Input: part model. Units: mm. Frame: model coordinates. Face numbers are marked on the shaded views. A direction names the side the tool comes from. Round coordinates to 2 decimals unless told otherwise and drop trailing zeros. Loops run counter-clockwise (first coordinate to the right, second up) from the corner with the lowest first, then second, coordinate; pieces in that order, holes last. Notation, with made-up numbers: (18, -21.75) -> (57, -21.75) arc R16 ccw to (57, -2.75) -> close; hole circle Ø5 at (78, -1). An arc over 180 degrees is marked (long way). Answer as a JSON object with one key per item and string values.
```python
from build123d import *

# Parameters (mm, degrees)
SKETCH1_R               = 7
SKETCH1_R_2             = 4.05
BOSS_EXTRUDE1_DEPTH     = 15
BOSS_EXTRUDE2_START     = -15
SKETCH1_3_R             = 7
SKETCH1_3_R_2           = 4.05
SKETCH1_3_R_3           = 1.7
BOSS_EXTRUDE2_DEPTH     = 15
SKETCH3_W               = 6
SKETCH3_H               = 3
CUT_EXTRUDE2_DEPTH      = 11
BOSS_EXTRUDE3_DEPTH     = 11
BOSS_EXTRUDE4_START     = -11
BOSS_EXTRUDE4_DEPTH     = 11
CUT_EXTRUDE1_DEPTH      = 20.874606914
CUT_EXTRUDE1_DEPTH_BACK = 20.874606914
SKETCH2_R               = 1.5


with BuildPart() as part:
    # Sketch1 → Boss-Extrude1 (new body)
    with BuildSketch(Plane(origin=(0, 0, 0), x_dir=(1, 0, 0), z_dir=(0, 1, 0))):
        with Locations(Location((0, 0, 0), (0, 0, 270))):
            Circle(SKETCH1_R)
        with Locations(Location((0, 0, 0), (0, 0, 270))):
            Circle(SKETCH1_R_2, mode=Mode.SUBTRACT)
    extrude(amount=BOSS_EXTRUDE1_DEPTH)

    # Sketch1_3 → Boss-Extrude2 (add)
    # profile 1 of 2: a face of its own
    with BuildSketch(Plane(origin=(0, 0, 0), x_dir=(1, 0, 0), z_dir=(0, 1, 0)).offset(BOSS_EXTRUDE2_START)):
        with Locations(Location((0, 0, 0), (0, 0, 270))):
            Circle(SKETCH1_3_R)
        with Locations(Location((0, 0, 0), (0, 0, 270))):
            Circle(SKETCH1_3_R_2, mode=Mode.SUBTRACT)
    # profile 2 of 2: a face of its own
    with BuildSketch(Plane(origin=(0, 0, 0), x_dir=(1, 0, 0), z_dir=(0, 1, 0)).offset(BOSS_EXTRUDE2_START)):
        with Locations(Location((0, 0, 0), (0, 0, 270))):
            Circle(SKETCH1_3_R_2)
        with Locations(Location((0, 0, 0), (0, 0, 270))):
            Circle(SKETCH1_3_R_3, mode=Mode.SUBTRACT)
    extrude(amount=BOSS_EXTRUDE2_DEPTH)

    # Sketch3 → Cut-Extrude2 (cut)
    with BuildSketch(Plane.XZ.offset(15)):
        with Locations((0, 5)):
            Rectangle(SKETCH3_W, SKETCH3_H)
    extrude(amount=-CUT_EXTRUDE2_DEPTH, mode=Mode.SUBTRACT)

    # Sketch3_3 → Boss-Extrude3 (add)
    with BuildSketch(Plane.XZ.offset(15)):
        with BuildLine():
            Line((-3, 6.32455532), (-3, 6.5))
            Line((-3, 6.5), (-2.598076211, 6.5))
            ThreePointArc((-2.598076211, 6.5), (0, 7), (2.598076211, 6.5))
            Line((2.598076211, 6.5), (3, 6.5))
            Line((3, 6.5), (3, 6.32455532))
            ThreePointArc((3, 6.32455532), (4.063012013, 5.700169593), (5, 4.898979486))
            Line((5, 4.898979486), (5, 8.5))
            Line((5, 8.5), (-5, 8.5))
            Line((-5, 8.5), (-5, 4.898979486))
            ThreePointArc((-5, 4.898979486), (-4.063012013, 5.700169593), (-3, 6.32455532))
        make_face()
    extrude(amount=-BOSS_EXTRUDE3_DEPTH)

    # Sketch4 → Boss-Extrude4 (add)
    with BuildSketch(Plane(origin=(0, 15, 0), x_dir=(1, 0, 0), z_dir=(0, 1, 0)).offset(BOSS_EXTRUDE4_START)):
        with BuildLine():
            Line((-3.605551275, -6), (-3, -6))
            Line((-3, -6), (3, -6))
            Line((3, -6), (3.605551275, -6))
            ThreePointArc((3.605551275, -6), (4.337849667, -5.4939112), (5, -4.898979486))
            Line((5, -4.898979486), (-5, -4.898979486))
            ThreePointArc((-5, -4.898979486), (-4.337849667, -5.4939112), (-3.605551275, -6))
        make_face()
        with BuildLine():
            Line((-3, -9), (-3, -6.32455532))
            ThreePointArc((-3, -6.32455532), (-3.306759887, -6.169711423), (-3.605551275, -6))
            Line((-3.605551275, -6), (-5, -6))
            Line((-5, -6), (-5, -11))
            Line((-5, -11), (5, -11))
            Line((5, -11), (5, -6))
            Line((5, -6), (3.605551275, -6))
            ThreePointArc((3.605551275, -6), (3.306759887, -6.169711423), (3, -6.32455532))
            Line((3, -6.32455532), (3, -9))
            Line((3, -9), (-3, -9))
        make_face()
        with BuildLine():
            Line((-5, -6), (-3.605551275, -6))
            ThreePointArc((-3.605551275, -6), (-4.337849667, -5.4939112), (-5, -4.898979486))
            Line((-5, -4.898979486), (-5, -6))
        make_face()
        with BuildLine():
            ThreePointArc((5, -4.898979486), (4.337849667, -5.4939112), (3.605551275, -6))
            Line((3.605551275, -6), (5, -6))
            Line((5, -6), (5, -4.898979486))
        make_face()
    extrude(amount=BOSS_EXTRUDE4_DEPTH)

    # Sketch2 → Cut-Extrude1 (cut, two sides: drawn at the far end of the back side and taken through both)
    with BuildSketch(Plane.XY.offset(-CUT_EXTRUDE1_DEPTH_BACK)):
        with Locations((0, 8)):
            Circle(SKETCH2_R)
        with Locations(Location((0, -8, 0), (0, 0, 180))):
            Circle(SKETCH2_R)
    extrude(amount=CUT_EXTRUDE1_DEPTH + CUT_EXTRUDE1_DEPTH_BACK, mode=Mode.SUBTRACT)


solid = part.part
```
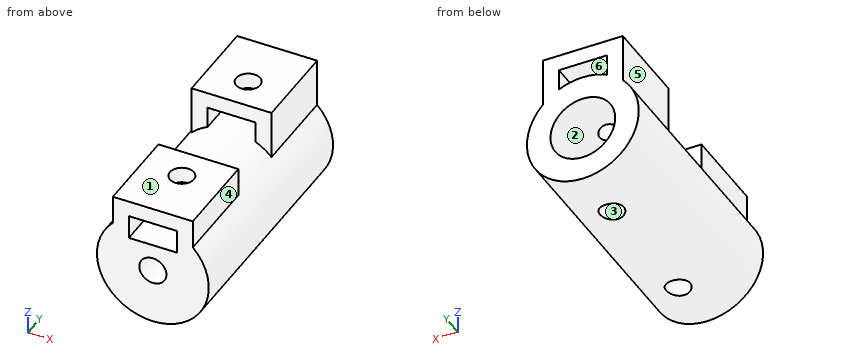
1) Section B-B, the plane z = 3. Output: boundary loops of the cut face in (x, y), plus the area to 3 significant figures.
Output:
{"outline": "(-6.32, -15) -> (6.32, -15) -> (6.32, 15) -> (2.72, 15) -> (2.72, 0) -> (-2.72, 0) -> (-2.72, 15) -> (-6.32, 15) -> close; hole circle Ø3 at (0, -8)", "area": "291 mm^2"}
2) Ray query, probe 1 along Y at (x, z) = (0, -6); probe 2 along X at (y, z) = (-8.5, 6); probe 3 along X at (y, z) = (-4.5, 0). Return the intervals inside material, ascending.
Output:
{"probe 1": "y = -15 to -9.5, -6.5 to 6.5, 9.5 to 15", "probe 2": "x = -5 to -3, 3 to 5", "probe 3": "x = -7 to -1.7, 1.7 to 7"}
3) Section A-A, the plane y = -5.5. Output: boundary loops of the cut face in (x, z), plus the area to 3 significant figures.
Output:
{"outline": "(-5, 4.9) arc R7 ccw (long way) to (5, 4.9) -> (5, 8.5) -> (-5, 8.5) -> close; hole (-3, 3.5) -> (3, 3.5) -> (3, 6.5) -> (-3, 6.5) -> close; hole circle Ø3.4 at (0, 0)", "area": "148 mm^2"}
4) Contact query for flat-ended pins moving along their axis: P1, Ø5, axis at x = -1, y = 11, coming from the -Z side; P2, Ø5, axis at x = -1, y = -9, coming from the +Z side; P3, Ø5, axis at y = 3.5, z = 5, coming from the -X side; P4, Ø1, axis at x = 4, y = 9.5, coming from the -Z side. Output: stop coordinate, or through.
Output:
{"P1": "stops at z = -7", "P2": "stops at z = 8.5", "P3": "stops at x = -6.54", "P4": "stops at z = -6.06"}
5) Section D-D, the plane x = 0. Count the separate pieces of the cut face and the enclosed holes in it, plus the area to 3 significant figures.
Output:
{"separate pieces": "9", "enclosed holes": "0", "area": "202 mm^2"}
6) Reachability of the marked faces 4, 5 and 6 from +Z, -Z, +X, -X, +Y, -Y: full face, straight path, thin tool, end or side. Return the list, or none.
Output:
{"face 4": "+Z, +X, +Y, -Y", "face 5": "+Z, -X, +Y, -Y", "face 6": "+Y, -Y"}
7) Draft query along Z for the marked faces 1, 2 and 3. Return one class per face: +Z half, -Z half, draft (parallel to the pull), parting line (faces both ways), or undercut.
Output:
{"face 1": "+Z half", "face 2": "undercut", "face 3": "draft"}
8) Section C-C, the plane y = 8. Output: boundary loops of the cut face in (x, z), plus the area to 3 significant figures.
Output:
{"outline": "(-5, 4.9) arc R7 ccw to (-1.5, -6.84) -> (-1.5, -3.76) arc R4.05 cw to (-1.5, 3.76) -> (-1.5, 6.84) arc R7 ccw to (-3, 6.32) -> (-3, 9) -> (-1.5, 9) -> (-1.5, 11) -> (-5, 11) -> close; (1.5, -6.84) arc R7 ccw to (5, 4.9) -> (5, 11) -> (1.5, 11) -> (1.5, 9) -> (3, 9) -> (3, 6.32) arc R7 ccw to (1.5, 6.84) -> (1.5, 3.76) arc R4.05 cw to (1.5, -3.76) -> close", "area": "112 mm^2"}
